Autodesk Inventor part; units mm, degrees
ref_plane "작업 평면1" through (-10.75, 2, 0) normal (0, 1, 0) x (1, 0, 0)
ref_plane "YZ Plane" through (0, 0, 0) normal (1, 0, 0) x (0, 1, 0)
ref_plane "XZ Plane" through (0, 0, 0) normal (0, 1, 0) x (-1, 0, 0)
sketch "스케치1" plane through (0, 0, 0) normal (0, 0, 1) x (1, 0, 0)
  line L0 (-12.75, -12) -> (12.75, -12)
  line L1 (12.75, -12) -> (12.75, 12)
  line L2 (12.75, 12) -> (-12.75, 12)
  line L3 (-12.75, 12) -> (-12.75, -12)
  line L4 (-12.75, -12) -> (12.75, 12) construction
  line L5 (12.75, -12) -> (-12.75, 12) construction
  line L6 (-4.25, 2.8) -> (4.25, 2.8)
  line L7 (4.25, 2.8) -> (4.25, -5.7)
  line L8 (4.25, -5.7) -> (-4.25, -5.7)
  line L9 (-4.25, -5.7) -> (-4.25, 2.8)
  line L10 (-4.25, 2.8) -> (4.25, -5.7) construction
  line L11 (4.25, 2.8) -> (-4.25, -5.7) construction
  line L12 (-5.95, 9.8) -> (3.25, 9.8)
  line L13 (3.25, 9.8) -> (3.25, 5.8)
  line L14 (3.25, 5.8) -> (-5.95, 5.8)
  line L15 (-5.95, 5.8) -> (-5.95, 9.8)
  line L16 (3.25, 9.8) -> (-3.85, 9.8)
  line L17 (-3.85, 9.8) -> (-3.85, 2.8)
  line L18 (-3.85, 2.8) -> (3.25, 2.8)
  line L19 (3.25, 2.8) -> (3.25, 9.8)
  circle A0 centre (-10.75, 10) radius 1
  point P0 (0, 0)
  point P1 (0, -1.45)
  point P2 (3.25, 2.8)
  point P3 (-3.85, 5.8)
  point P4 (0, -1.45)
  point P5 (0, 0)
  dimension "d0" = 25.5
  dimension "d1" = 24
  dimension "d2" = 8.5
  dimension "d3" = 8.5
  dimension "d4" = 17.7
  dimension "d5" = 1
  dimension "d6" = 7.1
  dimension "d7" = 4
  dimension "d8" = 7
  dimension "d9" = 9.2
  dimension "d10" = 2
  dimension "d11" = 2
  dimension "d12" = 2
extrude "돌출1" add sketch "스케치1" against normal blind 1 contours L3 L2 L1 L0 | L6 L7 L8 L9 | L17 L14 L19 L6 | L17 L12 L13 L14 | L14 L15 L12 L17 | A0
extrude "돌출2" cut sketch "스케치1" against normal blind 1 contours A0
extrude "돌출3" add sketch "스케치1" along normal blind 1.3 contours L17 L14 L19 L6 | L17 L12 L13 L14 | L14 L15 L12 L17
fillet "모깎기1" radius 2 4 edges at (-12.75, 12, -0.5) (-12.75, -12, -0.5) (12.75, -12, -0.5) (12.75, 12, -0.5)
mirror "미러3" about plane through (0, 0, 0) normal (1, 0, 0) of "돌출2"
pattern_linear "직사각형 패턴1" count 2 spacing 12 along (0, -1, 0) of "돌출2", "미러3"
sketch "스케치2" plane through (0, 0, 0) normal (0, 0, 1) x (1, 0, 0)
  point P0 (0, 0)
sketch "스케치4" plane through (0, 0, 0) normal (0, 0, 1) x (1, 0, 0)
  circle A0 centre (-10.75, 10) radius 1
  arc A1 (-10.75, 12) -> (-12.75, 10) centre (-10.75, 10) ccw
  circle A2 centre (-10.75, 10) radius 2
  circle A3 centre (10.75, 10) radius 1
  line L0 (10.75, 12) -> (-10.75, 12)
  circle A4 centre (10.75, 10) radius 2
  circle A5 centre (10.75, -2) radius 1
  circle A6 centre (10.75, -2) radius 2
  circle A7 centre (-10.75, -2) radius 2
  line L1 (-12.75, 10) -> (-12.75, -10)
  circle A8 centre (-10.75, -2) radius 1
  point P0 (0, 0)
  point P1 (-12.75, 10)
extrude "돌출7" add sketch "스케치4" along normal blind 0.1
sketch "스케치5" plane through (0, 0, -1) normal (0, 0, -1) x (-1, 0, 0)
  line L0 (10.75, -12) -> (-10.75, -12)
  line L1 (-10.5, -6.3) -> (10.5, -6.3)
  line L2 (10.5, -6.3) -> (10.5, -12)
  line L3 (10.5, -12) -> (-10.5, -12)
  line L4 (-10.5, -12) -> (-10.5, -6.3)
  point P0 (0, 0)
  point P1 (0, -12)
  dimension "d36" = 21
  dimension "d37" = 5.7
extrude "돌출8" add sketch "스케치5" along normal blind 2.6
sketch "스케치6" plane through (-10.75, -12, 0) normal (0, -1, 0) x (1, 0, 0)
  line L0 (21.25, -1) -> (0.25, -1)
  line L1 (0.25, -1) -> (0.25, -3.6)
  line L2 (21.25, -1) -> (0.25, -1)
  line L3 (0.25, -1) -> (0.25, -1.2)
  line L4 (0.25, -1.2) -> (21.25, -1.2)
  line L5 (21.25, -1.2) -> (21.25, -1)
  point P0 (10.75, 0)
  dimension "d40" = 0.2
extrude "돌출9" cut sketch "스케치6" against normal blind 2
ref_plane "작업 평면1" through (-10.75, 2, 0) normal (0, 1, 0) x (1, 0, 0)
sketch "스케치7" plane through (-10.75, 2, 0) normal (0, 1, 0) x (1, 0, 0)
  line L0 (14, 0) -> (6.9, 0)
  line L1 (6.9, 0) -> (14, 0)
  line L2 (14, 0) -> (14, -3.5)
  line L3 (14, -3.5) -> (6.9, -3.5)
  line L4 (6.9, -3.5) -> (6.9, 0)
  line L5 (6.2, -12) -> (14.7, -12)
  line L6 (14.7, -12) -> (14.7, -3.5)
  line L7 (14.7, -3.5) -> (6.2, -3.5)
  line L8 (6.2, -3.5) -> (6.2, -12)
  line L9 (6.2, -12) -> (14.7, -3.5) construction
  line L10 (14.7, -12) -> (6.2, -3.5) construction
  point P0 (10.75, 0)
  point P1 (10.45, -7.75)
  point P2 (10.45, -3.5)
  dimension "d45" = 12
  dimension "d46" = 8.5
  dimension "d47" = 8.5
extrude "돌출10" add sketch "스케치7" along normal blind 1 contours L2 L3 L4 L0
extrude "돌출11" add sketch "스케치7" along normal blind 2 contours L7 L6 L5 L8 L3
sketch "스케치8" plane through (-10.75, 4, 0) normal (0, 1, 0) x (1, 0, 0)
  line L0 (6.2, -12) -> (14.7, -12)
  line L1 (10.45, -12) -> (10.45, -3.5) construction
  line L2 (6.9, -3.5) -> (14, -3.5)
  circle A0 centre (10.45, -7.75) radius 4
  point P0 (10.75, 0)
  dimension "d52" = 8
extrude "돌출12" add sketch "스케치8" along normal blind 1
properties part number "RasCamera"
CAD build for the part. Positions are in the model's coordinates, mm. A direction names the side the tool comes from. Coordinates: 2 decimals unless noted, no trailing zeros. Write each loop counter-clockwise with the first axis right and the second up, starting at its lowest first coordinate (ties: lowest second). Pieces come first, ordered by that corner, then holes.
(1) Cut at A-A, the plane y = -8.75. List the corners of the cut face in (x, z), and give its area (3 significant figures).
(2) Cut at D-D, the plane x = -0.3. List the corners of the cut face in (y, z).
(3) Cut at C-C, the plane x = -5.5. List the corners of the cut face in (y, z).
(4) 3-axis set-ups, long thin cutter, end or side, ignore diameter. For faces 1 (the face through (0, 5, 8)), 2 (the face through (10.5, -9, -2)), 3 (the face through (0, -11, -1.2)), 4 (the face through (-4.55, 3, 8)), 5 (the face through (-5, 5.8, 1)): which of +Z, -Z, +X, -X, +Y, -Y reach the whole face in a straight line?
(5) Flat gauge pins, fed straight in: pin 1 (3 mm diameter, centred on x = 1, z = -2, fed in from +Y); pin 2 (1 mm diameter, centred on y = 3, z = 6.5, fed in from -X); pin 3 (10 mm diameter, centred on x = -5, y = 1, fed in from -Z); pin 4 (1 mm diameter, centred on y = 2.5, z = 8, fed in from +X). Where does each tip first touch, or does it go through?
(6) Cut at B-B, the plane z = 7.75. List the corners of the cut face in (x, y), and give its area (3 significant figures).
(7) Drill centre lines: probe 1 along Y at (x, z) = (-10.75, -0.35); probe 2 along Z at (x, y) = (-5.25, -5.25); probe 3 along X at (y, z) = (3, 10.25). Where is each one in solid material? Low to high.
Geometry says:
1. outline: (-12.75, -1) - (-10.5, -1) - (-10.5, -3.6) - (10.5, -3.6) - (10.5, -1) - (12.75, -1) - (12.75, 0) - (-12.75, 0) - close
1. area: 80.1 mm2
2. outline: (-12, -3.6) - (-6.3, -3.6) - (-6.3, -1) - (12, -1) - (12, 0) - (9.8, 0) - (9.8, 1.3) - (3, 1.3) - (3, 3.5) - (4, 3.5) - (4, 3.75) - (5, 3.75) - (5, 11.75) - (4, 11.75) - (4, 12) - (2, 12) - (2, 0) - (-12, 0) - (-12, -1) - (-10, -1) - (-10, -1.2) - (-12, -1.2) - close
3. outline: (-12, -3.6) - (-6.3, -3.6) - (-6.3, -1) - (12, -1) - (12, 0) - (9.8, 0) - (9.8, 1.3) - (5.8, 1.3) - (5.8, 0) - (-12, 0) - (-12, -1) - (-10, -1) - (-10, -1.2) - (-12, -1.2) - close
4. face 1: +Z, +X, -X, +Y
4. face 2: -Z, +X, +Y, -Y
4. face 3: +X, -X, -Y
4. face 4: +Z, -X, +Y, -Y
4. face 5: +Z, -X, -Y
5. pin 1: stops at y = 12
5. pin 2: stops at x = -4.55
5. pin 3: stops at z = -1
5. pin 4: stops at x = 3.95
6. outline: (-4.55, 2) - (3.95, 2) - (3.95, 4) - (3.7, 4) - (3.7, 5) - (-4.3, 5) - (-4.3, 4) - (-4.55, 4) - close
6. area: 25.0 mm2
7. probe 1: y = -12 to -3, -1 to 9, 11 to 12
7. probe 2: z = -1 to 0
7. probe 3: x = -4.55 to 3.95
